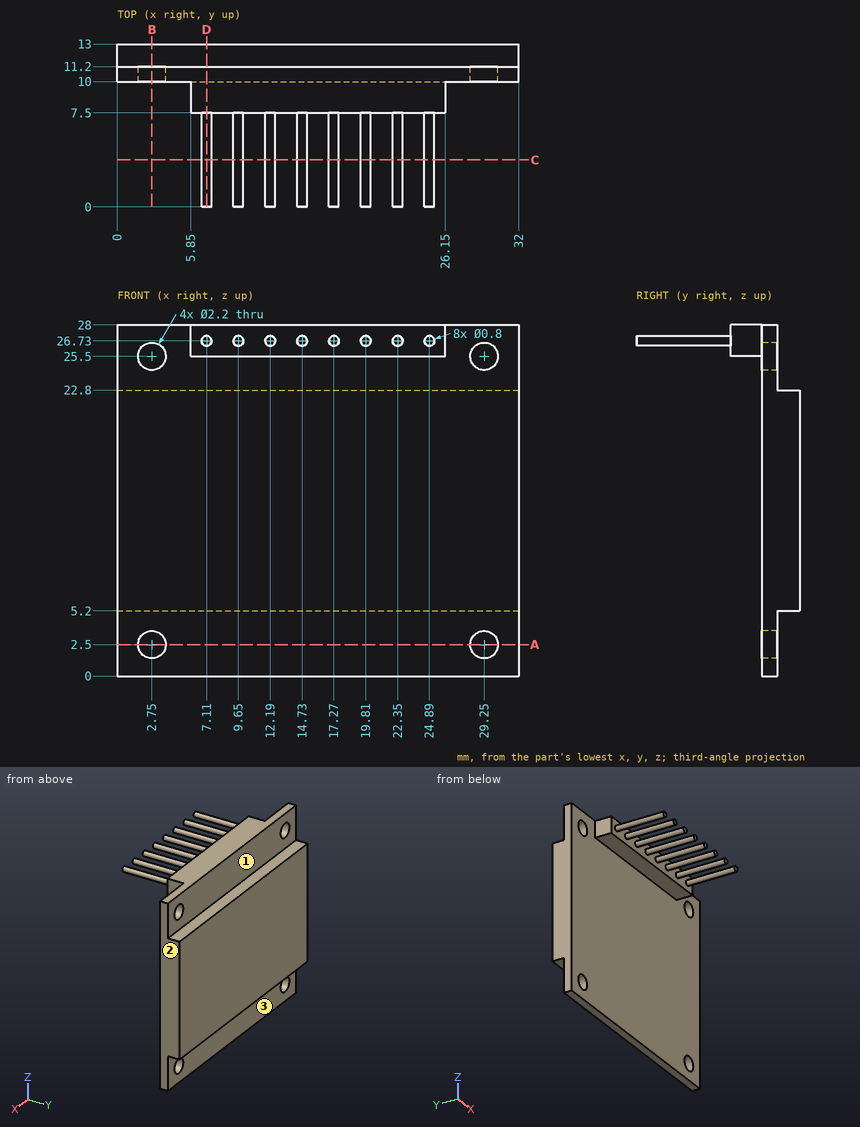
Here's the drawing with two shaded views (mm, measured from the low corner). I have some questions. A direction names the side the tool comes from. Give positions to 0.01 mm unless a question says otherwise; leave off trailing zeros. Write each loop counter-clockwise with the first axis right and the second up, starting at its lowest first coordinate (ties: lowest second). Pieces come first, ordered by that corner, then holes. Notation, with made-up numbers: (60, -37.75) - (111, -37.75) arc R30 ccw to (111, -6.75) - close; hole circle Ø5 at (-16, 38). An arc over 180 degrees is marked (long way). One line per item, written item: value. Start each with the question number.
Item 1: Imagine slicing it at A-A, the plane z = 2.5. List the corners of the cut face in (x, y) for me.
Item 2: Please list where these lines run through material, in increasing order: line 1 (X direction, y = 10.85, z = 2.5); line 2 (Y direction, x = 8, z = 13); line 3 (Y direction, x = 15, z = 24.5). Write a range as from..to.
Item 3: Imagine slicing it at D-D, the plane x = 7.11. List the corners of the cut face in (y, z) for me, and give its area (3 significant figures).
Item 4: Imagine slicing it at B-B, the plane x = 2.75. List the corners of the cut face in (y, z) for me, and give its area (3 significant figures).
Item 5: Which directions (+Z, -Z, +X, -X, +Y, -Y) give clear straight access to the entire face, cutting with the end or side of a thin tool? Please do the marked faces 1, 2 and 3.
Item 6: I'm going to push flat-ended pins straight in: pin 1 (4 mm diameter, centred on x = 29, z = 3, fed in from +Y); pin 2 (1.8 mm diameter, centred on x = 29.25, z = 2.5, fed in from +Y); pin 3 (2 mm diameter, centred on x = 17.5, y = 8.5, fed in from -Z); pin 4 (0.9 mm diameter, centred on x = 8, y = 12.5, fed in from +Z). Where does each tip first touch, or does it pass through?
Item 7: Imagine slicing it at C-C, the plane y = 3.75. List the corners of the cut face in (x, z) for me, and give its area (3 significant figures).
Geometry says:
1. outline: (0, 10) - (1.65, 10) - (1.65, 11.2) - (0, 11.2) - close; (3.85, 10) - (28.15, 10) - (28.15, 11.2) - (3.85, 11.2) - close; (30.35, 10) - (32, 10) - (32, 11.2) - (30.35, 11.2) - close
2. line 1: 0..1.65, 3.85..28.15, 30.35..32
2. line 2: 10..13
2. line 3: 10..11.2
3. outline: (0, 26.33) - (7.5, 26.33) - (7.5, 25.5) - (10, 25.5) - (10, 0) - (11.2, 0) - (11.2, 5.2) - (13, 5.2) - (13, 22.8) - (11.2, 22.8) - (11.2, 28) - (7.5, 28) - (7.5, 27.13) - (0, 27.13) - close
3. area: 77.5 mm^2
4. outline: (10, 0) - (11.2, 0) - (11.2, 1.4) - (10, 1.4) - close; (10, 3.6) - (11.2, 3.6) - (11.2, 5.2) - (13, 5.2) - (13, 22.8) - (11.2, 22.8) - (11.2, 24.4) - (10, 24.4) - close; (10, 26.6) - (11.2, 26.6) - (11.2, 28) - (10, 28) - close
4. area: 60.0 mm^2
5. face 1: +Z, +X, -X, +Y
5. face 2: +Z, -Z, +X, +Y, -Y
5. face 3: -Z, +X, -X, +Y
6. pin 1: y = 11.2
6. pin 2: through
6. pin 3: z = 25.5
6. pin 4: z = 22.8
7. outline: circle Ø0.8 at (7.11, 26.73); circle Ø0.8 at (9.65, 26.73); circle Ø0.8 at (12.19, 26.73); circle Ø0.8 at (14.73, 26.73); circle Ø0.8 at (17.27, 26.73); circle Ø0.8 at (19.81, 26.73); circle Ø0.8 at (22.35, 26.73); circle Ø0.8 at (24.89, 26.73)
7. area: 4.02 mm^2
